```python
from build123d import *

# Parameters (mm, degrees)
BOSS_EXTRUDE3_DEPTH = 50
SKETCH4_R           = 25
BOSS_EXTRUDE4_DEPTH = 1100
SKETCH5_R           = 15
CUT_EXTRUDE1_DEPTH  = 161


with BuildPart() as part:
    # Sketch1 → Boss-Extrude3 (new body, symmetric)
    with BuildSketch(Plane(origin=(0, 0, 0), x_dir=(1, 0, 0), z_dir=(0, 1, 0))):
        Polygon((5, 150), (5, 5), (155, 5), (155, 150), (160, 150), (160, 0), (0, 0), (0, 150), align=None)
    extrude(amount=BOSS_EXTRUDE3_DEPTH, both=True)

    # Sketch4 → Boss-Extrude4 (add)
    with BuildSketch(Plane.XY):
        with Locations((80, 0)):
            Circle(SKETCH4_R)
    extrude(amount=BOSS_EXTRUDE4_DEPTH)

    # Sketch5 → Cut-Extrude1 (cut, through all)
    with BuildSketch(Plane(origin=(160, 0, 0), x_dir=(0, 0, -1), z_dir=(1, 0, 0))):
        with Locations((125, 0)):
            Circle(SKETCH5_R)
    extrude(amount=-CUT_EXTRUDE1_DEPTH, mode=Mode.SUBTRACT)


solid = part.part
```
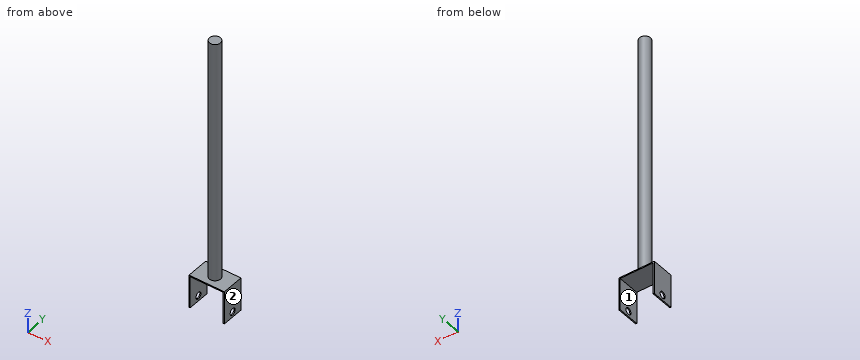
CAD build for the part. Positions are in the model's coordinates, mm. Face numbers are marked on the shaded views. A direction names the side the tool comes from. Coordinates: 2 decimals unless noted, no trailing zeros. Write each loop counter-clockwise with the first axis right and the second up, starting at its lowest first coordinate (ties: lowest second). Pieces come first, ordered by that corner, then holes.
(1) Cut at A-A, the plane y = 0. List the corners of the cut face in (x, z).
(2) Cut at D-D, the plane z = 256.5. List the corners of the cut face in (x, y).
(3) 3-axis set-ups, long thin cutter, end or side, ignore diameter. For the marked faces 1 and 2: which of +Z, -Z, +X, -X, +Y, -Y reach the whole face in a straight line?
(4) Flat gauge pins, fed straight in: pin 1 (4 mm diameter, centred on y = -4.5, z = 112, fed in from +X); pin 2 (5 mm diameter, centred on x = 65.5, z = 621, fed in from -Y); pin 3 (8 mm diameter, centred on y = 5.5, z = 905, fed in from -X); pin 4 (4 mm diameter, centred on x = 107.5, z = 404, fed in from -Y). Where does each tip first touch, or does it go through?
(5) Cut at C-C, the plane x = 80. List the corners of the cut face in (y, z), and give its area (3 significant figures).
(6) Drill centre lines: probe 1 along X at (y, z) = (14, -81.5); probe 2 along Y at (x, z) = (2, -125); probe 3 along Z at (x, y) = (118, -29). Where is each one in solid material? Low to high.
(7) Cut at B-B, the plane z = -125. List the corners of the cut face in (x, y), and give its area (3 significant figures).
Geometry says:
1. outline: (0, -150) - (5, -150) - (5, -140) - (0, -140) - close; (0, -110) - (5, -110) - (5, -5) - (155, -5) - (155, -110) - (160, -110) - (160, 0) - (105, 0) - (105, 1100) - (55, 1100) - (55, 0) - (0, 0) - close; (155, -150) - (160, -150) - (160, -140) - (155, -140) - close
2. outline: circle Ø50 at (80, 0)
3. face 1: -Z, +Y, -Y
3. face 2: +Z, -Z, +X, +Y, -Y
4. pin 1: stops at x = 104.87
4. pin 2: stops at y = -21.93
4. pin 3: stops at x = 55.05
4. pin 4: passes through
5. outline: (-50, -5) - (50, -5) - (50, 0) - (25, 0) - (25, 1100) - (-25, 1100) - (-25, 0) - (-50, 0) - close
5. area: 55,500 mm2
6. probe 1: x = 0 to 5, 155 to 160
6. probe 2: y = -50 to -15, 15 to 50
6. probe 3: z = -5 to 0
7. outline: (0, -50) - (5, -50) - (5, -15) - (0, -15) - close; (0, 15) - (5, 15) - (5, 50) - (0, 50) - close; (155, -50) - (160, -50) - (160, -15) - (155, -15) - close; (155, 15) - (160, 15) - (160, 50) - (155, 50) - close
7. area: 700 mm2
